```python
from build123d import *

# Parameters (mm, degrees)
F0_W     = 8
F0_H     = 15
F1_DEPTH = 4.5
F2_W     = 0.9
F2_H     = 3.18
F2_W_2   = 1
F3_DEPTH = 2.7


# Not quite as in the source:
# - a feature names something its author has since deleted; it is built from what else it names


with BuildPart() as f1:
    # F0 (on Front) → F1 (new body)
    with BuildSketch(Plane.XZ):
        Polygon((-92.1357174787, 21.691892745), (-117.1357174787, 21.691892745), (-117.1357174787, -16.308107255), (-92.1357174787, -16.308107255), (-92.1357174787, 0.7088574011), (-94.8357174787, 0.7088574011), (-94.8357174787, 3.8888574011), (-92.1357174787, 3.8888574011), align=None)
        with Locations((-104.6122670679, 2.7691081924)):
            Rectangle(F0_W, F0_H, mode=Mode.SUBTRACT)
    extrude(amount=F1_DEPTH)

    # F2 (on face) → F3 (join)
    with BuildSketch(Plane.YZ.offset(-94.8357174787)):
        with Locations((-0.45, 2.2988574011)):
            Rectangle(F2_W, F2_H)
        with Locations((-4, 2.2988574011)):
            Rectangle(F2_W_2, F2_H)
    extrude(amount=F3_DEPTH)


solid = f1.part
```
Build history of the part. All positions in model axes, mm. A direction names the side the tool comes from. Give positions to 0.01 mm unless a question says otherwise; leave off trailing zeros. Loops run counter-clockwise (first coordinate to the right, second up) from the corner with the lowest first, then second, coordinate; pieces in that order, holes last. Notation, with made-up numbers: (67, 46) - (75, 46) arc R12 cw to (75, 54) - close; hole circle Ø6 at (82.5, 12.25). An arc over 180 degrees is marked (long way). Use a Markdown table: item, result.
(1) Band-saw the part on B-B (y = -2). Give the cut face in (x, z).
Taken from the geometry:
| item | result |
|---|---|
| outline | (-117.14, -16.31) - (-92.14, -16.31) - (-92.14, 0.71) - (-94.84, 0.71) - (-94.84, 3.89) - (-92.14, 3.89) - (-92.14, 21.69) - (-117.14, 21.69) - close; hole (-108.61, -4.73) - (-100.61, -4.73) - (-100.61, 10.27) - (-108.61, 10.27) - close |
(2) Band-saw the part on D-D (z = 3.5). Give the cut face in (x, y).
Taken from the geometry:
| item | result |
|---|---|
| outline | (-117.14, -4.5) - (-108.61, -4.5) - (-108.61, 0) - (-117.14, 0) - close; (-100.61, -4.5) - (-92.14, -4.5) - (-92.14, -3.5) - (-94.84, -3.5) - (-94.84, -0.9) - (-92.14, -0.9) - (-92.14, 0) - (-100.61, 0) - close |
(3) Wall check: line 1 along Z through (x, y) = (-106, -2.35); line 2 along X through (y, z) = (-3.4, 5); line 3 along Y through (x, z) = (-94.25, 2). Give the ranges that are in metal, low to high.
Taken from the geometry:
| item | result |
|---|---|
| line 1 | -16.31 to -4.73, 10.27 to 21.69 |
| line 2 | -117.14 to -108.61, -100.61 to -92.14 |
| line 3 | -4.5 to -3.5, -0.9 to 0 |
(4) Which spindle directions (+Z, -Z, +X, -X, +Y, -Y) get a long thin tool onto all of the face, cutting with end or side? Do faces 4 (the face through (-105, -2, -16.308)), 5 (the face through (-105, -2, -4.731)), 6 (the face through (-94, -0.9, 2)). Say none if no direction does.
Taken from the geometry:
| item | result |
|---|---|
| face 4 | -Z, +X, -X, +Y, -Y |
| face 5 | +Y, -Y |
| face 6 | +X |
(5) Band-saw the part on C-C (z = 9). Give the cut face in (x, y), and give its area (3 significant figures).
Taken from the geometry:
| item | result |
|---|---|
| outline | (-117.14, -4.5) - (-108.61, -4.5) - (-108.61, 0) - (-117.14, 0) - close; (-100.61, -4.5) - (-92.14, -4.5) - (-92.14, 0) - (-100.61, 0) - close |
| area | 76.5 mm2 |
(6) Pull direction Z, two halves, no side cores. Call faces 1 (the face through (-110, -4.5, 3)), 2 (the face through (-104, -2, 21.692)), 3 (the face through (-100.612, -2, 3)): +Z half, -Z half, draft (parallel to the pull), parting line (faces both ways), or undercut.
Taken from the geometry:
| item | result |
|---|---|
| face 1 | draft |
| face 2 | +Z half |
| face 3 | undercut |
(7) Band-saw the part on A-A (x = -106.25). Give the cut face in (y, z).
Taken from the geometry:
| item | result |
|---|---|
| outline | (-4.5, -16.31) - (0, -16.31) - (0, -4.73) - (-4.5, -4.73) - close; (-4.5, 10.27) - (0, 10.27) - (0, 21.69) - (-4.5, 21.69) - close |
(8) Drop a flat-ended pin along its axis: pin 1 Ø3 at (x, z) = (-93, 2) entering from +Y. Give the stop position or say it passes through.
Taken from the geometry:
| item | result |
|---|---|
| pin 1 | y = 0 |
